```python
from build123d import *

# Parameters (mm, degrees)
BOSS_EXTRUDE1_DEPTH = 1.016
SCALE1_SCALE        = 1.04
SKETCH2_R           = 1.11125
NEEDLE_CUT_DEPTH    = 15.98045747
TAB_CUT_DEPTH       = 15.98045747


with BuildPart() as part:
    # Sketch1 → Boss-Extrude1 (new body)
    with BuildSketch(Plane.XY):
        with BuildLine():
            ThreePointArc((7.62, -3.175), (8.255, 0), (7.62, 3.175))
            ThreePointArc((7.62, 3.175), (10.16, 0), (7.62, -3.175))
        make_face()
        with BuildLine():
            ThreePointArc((7.62, -3.175), (8.255, 0), (7.62, 3.175))
            ThreePointArc((7.62, 3.175), (0, 8.255), (-7.62, 3.175))
            ThreePointArc((-7.62, 3.175), (-8.255, 0), (-7.62, -3.175))
            ThreePointArc((-7.62, -3.175), (0, -8.255), (7.62, -3.175))
        make_face()
        with BuildLine():
            ThreePointArc((-7.62, 3.175), (-8.255, 0), (-7.62, -3.175))
            ThreePointArc((-7.62, -3.175), (-10.16, 0), (-7.62, 3.175))
        make_face()
        with BuildLine():
            ThreePointArc((3.175, 7.62), (0, 10.16), (-3.175, 7.62))
            ThreePointArc((-3.175, 7.62), (0, 8.255), (3.175, 7.62))
        make_face()
        with BuildLine():
            ThreePointArc((3.175, -7.62), (0, -8.255), (-3.175, -7.62))
            ThreePointArc((-3.175, -7.62), (0, -10.16), (3.175, -7.62))
        make_face()
    extrude(amount=BOSS_EXTRUDE1_DEPTH)


with BuildPart() as part_1:
    # Scale1: scaled about (0, 0, 0.508)
    add(part.part.scale(SCALE1_SCALE).moved(Location((0, 0, -0.02032))))

    # Sketch2 → Needle Cut (cut, through all)
    with BuildSketch(Plane.XY.offset(1.03632)):
        Circle(SKETCH2_R)
    extrude(amount=-NEEDLE_CUT_DEPTH, mode=Mode.SUBTRACT)

    # Sketch3 → Tab Cut (cut, through all)
    with BuildSketch(Plane.XY.offset(1.03632)):
        with BuildLine():
            ThreePointArc((-2.667, 6.832154423), (0, 7.33425), (2.667, 6.832154423))
            ThreePointArc((2.667, 6.832154423), (0, 8.284442607), (-2.667, 6.832154423))
        make_face()
        with BuildLine():
            ThreePointArc((6.832154423, 2.667), (7.207633164, 1.356925658), (7.33425, 0))
            ThreePointArc((7.33425, 0), (7.207633164, -1.356925658), (6.832154423, -2.667))
            ThreePointArc((6.832154423, -2.667), (8.284442607, 0), (6.832154423, 2.667))
        make_face()
        with BuildLine():
            ThreePointArc((-2.667, -6.832154423), (0, -8.284442607), (2.667, -6.832154423))
            ThreePointArc((2.667, -6.832154423), (0, -7.33425), (-2.667, -6.832154423))
        make_face()
        with BuildLine():
            ThreePointArc((-6.832154423, -2.667), (-7.33425, 0), (-6.832154423, 2.667))
            ThreePointArc((-6.832154423, 2.667), (-8.284442607, 0), (-6.832154423, -2.667))
        make_face()
    extrude(amount=-TAB_CUT_DEPTH, mode=Mode.SUBTRACT)


solid = part_1.part
```
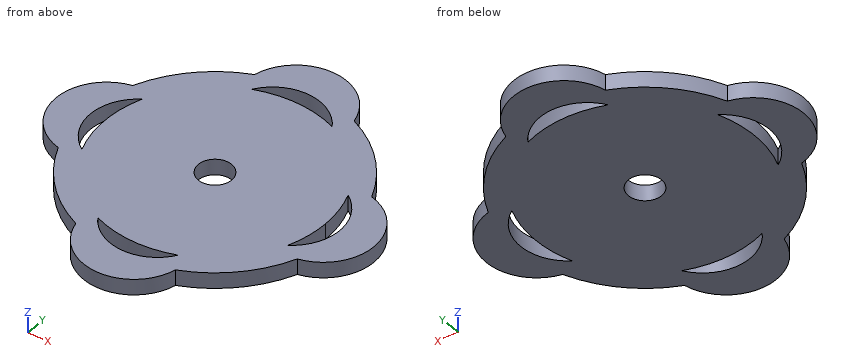
CAD build for the part. Positions are in the model's coordinates, mm. Give positions to 0.01 mm unless a question says otherwise; leave off trailing zeros. Loops run counter-clockwise (first coordinate to the right, second up) from the corner with the lowest first, then second, coordinate; pieces in that order, holes last. Notation, with made-up numbers: (40, 21) -> (60, 21) arc R20 cw to (60, 27) -> close; hole circle Ø9 at (50, -10). An arc over 180 degrees is marked (long way). Use a Markdown table: item, result.
1. Slice it at D-D (y = 6.25). List the corners of the cut face in (x, z).
Check result:
| item | result |
|---|---|
| outline | (-5.89, -0.02) -> (5.89, -0.02) -> (5.89, 1.04) -> (-5.89, 1.04) -> close |
2. Slice it at B-B (z = 0.3). Give the number of separate pieces and of enclosed holes in the cut face, plus the area to 3 significant figures.
Check result:
| item | result |
|---|---|
| separate pieces | 1 |
| enclosed holes | 5 |
| area | 253 mm^2 |
3. Wall check: L1, parallel to Y at x = -0.75, z = 0.3; L2, parallel to Y at x = 1.75, z = 0.2; L3, parallel to X at y = -2, z = 0.35. Give the ranges that are in metal, low to high. Write a range as [from, to].
Check result:
| item | result |
|---|---|
| L1 | y = [-10.48, -8.19], [-7.3, -0.82], [0.82, 7.3], [8.19, 10.48] |
| L2 | y = [-10.08, -7.76], [-7.12, 7.12], [7.76, 10.08] |
| L3 | x = [-9.91, -7.58], [-7.06, 7.06], [7.58, 9.91] |
4. Slice it at C-C (y = 1.5). List the corners of the cut face in (x, z), plus the area to 3 significant figures.
Check result:
| item | result |
|---|---|
| outline | (-10.22, -0.02) -> (-7.91, -0.02) -> (-7.91, 1.04) -> (-10.22, 1.04) -> close; (-7.18, -0.02) -> (7.18, -0.02) -> (7.18, 1.04) -> (-7.18, 1.04) -> close; (7.91, -0.02) -> (10.22, -0.02) -> (10.22, 1.04) -> (7.91, 1.04) -> close |
| area | 20.0 mm^2 |
5. Slice it at A-A (x = 0). List the corners of the cut face in (y, z).
Check result:
| item | result |
|---|---|
| outline | (-10.57, -0.02) -> (-8.28, -0.02) -> (-8.28, 1.04) -> (-10.57, 1.04) -> close; (-7.33, -0.02) -> (-1.11, -0.02) -> (-1.11, 1.04) -> (-7.33, 1.04) -> close; (1.11, -0.02) -> (7.33, -0.02) -> (7.33, 1.04) -> (1.11, 1.04) -> close; (8.28, -0.02) -> (10.57, -0.02) -> (10.57, 1.04) -> (8.28, 1.04) -> close |
